Autodesk Fusion 360 part; units mm, degrees
sketch "Schizzo1" plane through (0, 0, 0) normal (0, 0, 1) x (1, 0, 0)
  line L0 (20.7879, 45.3781) -> (88.2879, 45.3781)
  line L1 (88.2879, 45.3781) -> (88.2879, 5.3781)
  line L2 (88.2879, 5.3781) -> (20.7879, 5.3781)
  line L3 (20.7879, 5.3781) -> (20.7879, 45.3781)
  line L4 (20.7879, 45.3781) -> (16.7879, 45.3781)
  line L5 (16.7879, 45.3781) -> (16.7879, 5.3781)
  line L6 (16.7879, 5.3781) -> (20.7879, 5.3781)
  line L7 (20.7879, 5.3781) -> (20.7879, 45.3781)
  line L8 (54.5379, 45.3781) -> (54.5379, 5.3781) construction
  line L9 (88.2879, 25.3781) -> (20.7879, 25.3781) construction
  line L10 (92.2879, 45.3781) -> (92.2879, 5.3781)
  line L11 (88.2879, 5.3781) -> (88.2879, 45.3781)
  line L12 (92.2879, 5.3781) -> (88.2879, 5.3781)
  line L13 (88.2879, 45.3781) -> (92.2879, 45.3781)
  line L14 (79.5379, 10.3781) -> (29.5379, 10.3781) construction
  line L15 (29.5379, 10.3781) -> (29.5379, 40.3781) construction
  line L16 (29.5379, 40.3781) -> (79.5379, 40.3781) construction
  line L17 (79.5379, 40.3781) -> (79.5379, 10.3781) construction
  line L18 (79.5379, 10.3781) -> (29.5379, 40.3781) construction
  line L19 (29.5379, 10.3781) -> (79.5379, 40.3781) construction
  circle A0 centre (29.5379, 40.3781) radius 2.05
  circle A1 centre (79.5379, 40.3781) radius 2.05
  circle A2 centre (29.5379, 10.3781) radius 2.05
  circle A3 centre (79.5379, 10.3781) radius 2.05
  circle A4 centre (54.5379, 40.3781) radius 2.05
  circle A5 centre (54.5379, 10.3781) radius 2.05
  line L20 (16.7879, 5.3781) -> (23.7879, 5.3781)
  line L21 (23.7879, 5.3781) -> (23.7879, 3.3781)
  line L22 (23.7879, 3.3781) -> (16.7879, 3.3781)
  line L23 (16.7879, 3.3781) -> (16.7879, 5.3781)
  line L24 (16.7879, 45.3781) -> (23.7879, 45.3781)
  line L25 (23.7879, 47.3781) -> (16.7879, 47.3781)
  line L26 (23.7879, 45.3781) -> (23.7879, 47.3781)
  line L27 (16.7879, 47.3781) -> (16.7879, 45.3781)
  line L28 (92.2879, 45.3781) -> (85.2879, 45.3781)
  line L29 (92.2879, 5.3781) -> (85.2879, 5.3781)
  line L30 (85.2879, 3.3781) -> (92.2879, 3.3781)
  line L31 (85.2879, 5.3781) -> (85.2879, 3.3781)
  line L32 (92.2879, 3.3781) -> (92.2879, 5.3781)
  line L33 (85.2879, 47.3781) -> (92.2879, 47.3781)
  line L34 (85.2879, 45.3781) -> (85.2879, 47.3781)
  line L35 (92.2879, 47.3781) -> (92.2879, 45.3781)
  circle A6 centre (54.5379, 25.3781) radius 5
  line L36 (23.7879, 5.3781) -> (85.2879, 5.3781)
  line L37 (85.2879, 5.3781) -> (85.2879, 3.3781)
  line L38 (85.2879, 3.3781) -> (23.7879, 3.3781)
  line L39 (23.7879, 3.3781) -> (23.7879, 5.3781)
  line L40 (23.7879, 47.3781) -> (85.2879, 47.3781)
  line L41 (85.2879, 47.3781) -> (85.2879, 45.3781)
  line L42 (85.2879, 45.3781) -> (23.7879, 45.3781)
  line L43 (23.7879, 45.3781) -> (23.7879, 47.3781)
  point P0 (54.5379, 25.3781)
  dimension "d1" = 67.5
  dimension "d2" = 40
  dimension "d3" = 4
  dimension "d4" = 50
  dimension "d5" = 30
  dimension "d6" = 4.1
  dimension "d8" = 4.1
  dimension "d13" = 7
  dimension "d14" = 2
  dimension "d15" = 10
  dimension "d19" = 7
  dimension "d20" = 75.5
extrude "Estrusione1" add sketch "Schizzo1" along normal blind 6 contours L0 L1 L2 L3 L7 L11 L20 L24 L28 L29 L36 L42 | L0 L26 L34 L40 L41 L42 L43 | L2 L21 L31 L36 L37 L38 L39
extrude "Estrusione2" add sketch "Schizzo1" along normal blind 90 contours L0 L4 L24 L25 L26 L27 L43 | L3 L4 L5 L6 L7 L20 L24 | L2 L6 L20 L21 L22 L23 L39 | L0 L13 L28 L33 L34 L35 L41 | L1 L10 L11 L12 L13 L28 L29 | L2 L12 L29 L30 L31 L32 L37
extrude "Estrusione3" add sketch "Schizzo1" along normal blind 5 from surface at 6 contours L0 L26 L34 L40 L41 L42 L43 | L2 L21 L31 L36 L37 L38 L39
equation "d8 = d6"
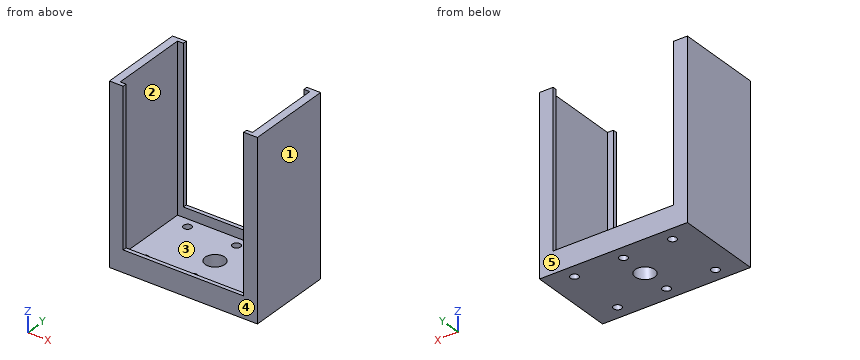
Geometry check sheet. Reference: the model listing, model coordinates, mm. Face numbers are marked on the shaded views. A direction names the side the tool comes from. Round coordinates to 2 decimals unless told otherwise and drop trailing zeros. Loops run counter-clockwise (first coordinate to the right, second up) from the corner with the lowest first, then second, coordinate; pieces in that order, holes last.
Item 1: Cross-section at C-C on y = 18. Record the boundary of the cut face in (x, z), then the cut area to 4 significant figures.
Item 2: Cross-section at B-B on x = 29.5. Record the boundary of the cut face in (y, z), then the cut area to 3 significant figures.
Item 3: Thickness scan on line 1 (X direction, y = 20.5, z = 71.5); line 2 (Y direction, x = 23, z = 43); line 3 (Z direction, x = 25, y = 20.5). Record the ranges inside material, lowest first.
Item 4: Gauge pin test, flat ends, axial feed: pin 1 (4.5 mm diameter, centred on x = 79.54, y = 10.38, fed in from +Z); pin 2 (0.6 mm diameter, centred on x = 66.5, y = 4, fed in from +Z). Record the tip position at first contact, or that the pin passes through.
Item 5: Mould release check, pull along Y, two halves, no side actions. Record for the marked faces 3, 4 and 5: pulls with the +Y half, pulls with the -Y half, needs draft (parallel to the pull), parting line crosses it, or undercut.
Item 6: Access from +Z, -Z, +X, -X, +Y, -Y to the whole of each face (thin tool, end or side, straight path). Record for the marked faces 1 and 2.
Item 7: Cross-section at A-A on z = 46. Record the boundary of the cut face in (x, y), then the cut area to 3 significant figures.
Item 8: Cross-section at D-D on x = 80. Record the boundary of the cut face in (y, z).
Answer sheet:
1. outline: (16.79, 0) - (92.29, 0) - (92.29, 90) - (88.29, 90) - (88.29, 6) - (20.79, 6) - (20.79, 90) - (16.79, 90) - close
1. area: 1,125 mm2
2. outline: (3.38, 0) - (8.33, 0) - (8.33, 6) - (5.38, 6) - (5.38, 11) - (3.38, 11) - close; (12.43, 0) - (38.33, 0) - (38.33, 6) - (12.43, 6) - close; (42.43, 0) - (47.38, 0) - (47.38, 11) - (45.38, 11) - (45.38, 6) - (42.43, 6) - close
2. area: 235 mm2
3. line 1: x = 16.79 to 20.79, 88.29 to 92.29
3. line 2: y = 3.38 to 5.38, 45.38 to 47.38
3. line 3: z = 0 to 6
4. pin 1: stops at z = 6
4. pin 2: stops at z = 11
5. face 3: undercut
5. face 4: pulls with the -Y half
5. face 5: pulls with the +Y half
6. face 1: +Z, -Z, +X, +Y, -Y
6. face 2: +Z
7. outline: (16.79, 3.38) - (23.79, 3.38) - (23.79, 5.38) - (20.79, 5.38) - (20.79, 45.38) - (23.79, 45.38) - (23.79, 47.38) - (16.79, 47.38) - close; (85.29, 3.38) - (92.29, 3.38) - (92.29, 47.38) - (85.29, 47.38) - (85.29, 45.38) - (88.29, 45.38) - (88.29, 5.38) - (85.29, 5.38) - close
7. area: 376 mm2
8. outline: (3.38, 0) - (8.38, 0) - (8.38, 6) - (5.38, 6) - (5.38, 11) - (3.38, 11) - close; (12.38, 0) - (38.38, 0) - (38.38, 6) - (12.38, 6) - close; (42.38, 0) - (47.38, 0) - (47.38, 11) - (45.38, 11) - (45.38, 6) - (42.38, 6) - close
